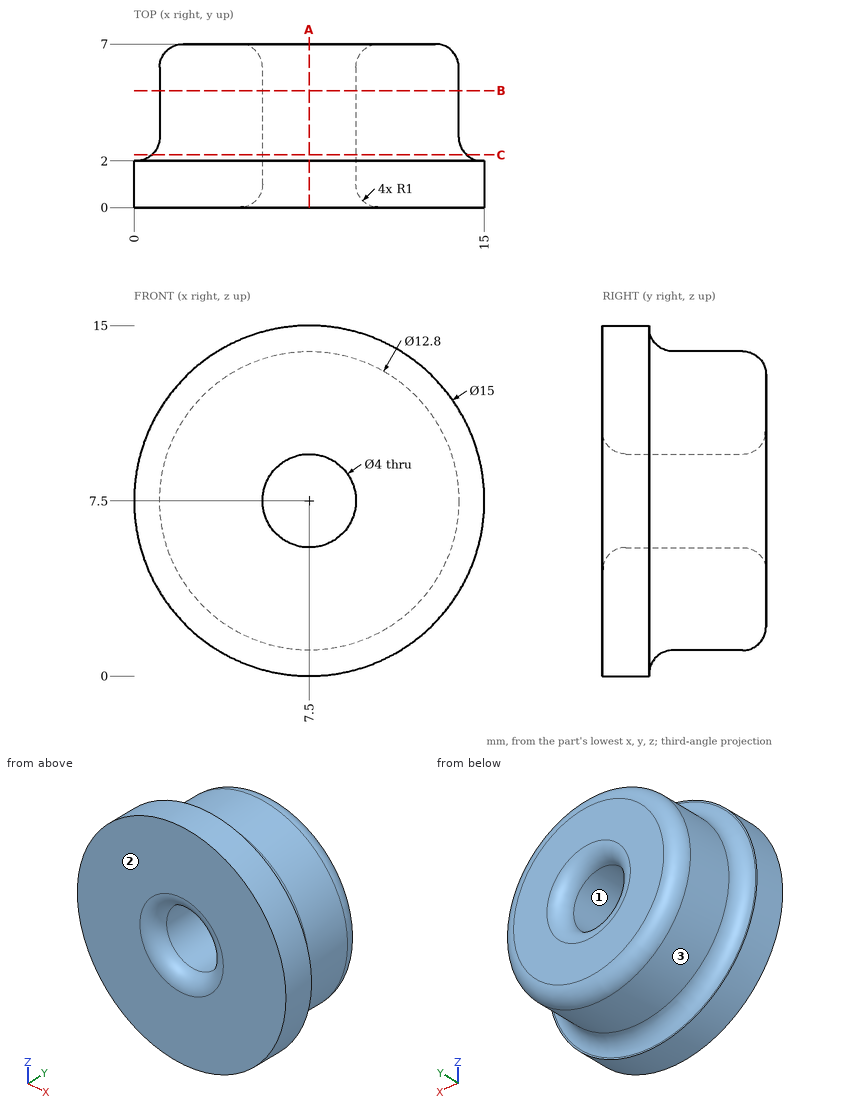
Source: three-view drawing plus pictorial views. Frame: mm from the lowest corner of the part. Give positions to 0.01 mm unless a question says otherwise; leave off trailing zeros. Order: outer loops, then holes, each group sorted by start corner. A loop starts at its lowest first (then second) coordinate and runs counter-clockwise, first axis right, second up. Notation, with made-up numbers: M 50.25,86 L 68.25,86 A10 cw 68.25,99 Z; hole C -7,6 d10. An arc over 180 degrees is marked long. Return JSON: item names as keys, results as strings.
Item 1: Ray query, probe 1 along X at (y, z) = (4.65, 7.5); probe 2 along X at (y, z) = (2.25, 7.5). Return the intervals inside material, ascending.
Solutions:
{"probe 1": "1.1 to 5.5, 9.5 to 13.9", "probe 2": "0.76 to 5.5, 9.5 to 14.24"}
Item 2: Pull-direction query (X, two-part tool) for the marked faces 1, 2 and 3; classes: +X half, -X half, draft (parallel to the pull), parting line (faces both ways), or undercut.
Solutions:
{"face 1": "undercut", "face 2": "draft", "face 3": "parting line"}
Item 3: Cut plane B-B (y = 5). Return loops of the section in (x, z).
Solutions:
{"outline": "C 7.5,7.5 d12.8; hole C 7.5,7.5 d4"}
Item 4: Cut plane C-C (y = 2.25). Return loops of the section in (x, z).
Solutions:
{"outline": "C 7.5,7.5 d13.48; hole C 7.5,7.5 d4"}
Item 5: First-contact query: P1, Ø4, axis at y = 5, z = 13, coming from the -X side; P2, Ø4, axis at x = 6, z = 8, coming from the +Y side; P3, Ø3, axis at x = 7.5, z = 7.5, coming from the -Y side. Flat tips, straight axial feed; report the tip coordinate or a pass-through.
Solutions:
{"P1": "x = 2.14", "P2": "y = 7", "P3": "through"}
Item 6: Cut plane A-A (x = 7.5). Return loops of the section in (y, z).
Solutions:
{"outline": "M 0,0 L 2,0 L 2,0.1 A1 cw 3,1.1 L 6,1.1 A1 ccw 7,2.1 L 7,4.5 A1 ccw 6,5.5 L 1,5.5 A1 ccw 0,4.5 Z; M 0,10.5 A1 ccw 1,9.5 L 6,9.5 A1 ccw 7,10.5 L 7,12.9 A1 ccw 6,13.9 L 3,13.9 A1 cw 2,14.9 L 2,15 L 0,15 Z"}
